Source: CAD feature listing. Evaluate the final solid. Frame: model axes, mm. Coordinates: 2 decimals unless noted, no trailing zeros. Write each loop counter-clockwise with the first axis right and the second up, starting at its lowest first coordinate (ties: lowest second). Pieces come first, ordered by that corner, then holes. Notation, with made-up numbers: M 2,-29.75 L 44,-29.75 A17 ccw 44,-1.75 Z; hole C -26.5,31.25 d10. An arc over 180 degrees is marked long. One line per item, written item: value. Start each with the question number.
Item 1: Pin query (flat end, axial travel): P1, Ø1.5, axis at x = 6.25, z = -0.5, coming from the +Y side. Return the tip coordinate at first contact, or that it passes through.
Item 2: Mould query, pull axis Y, two halves, no side actions, for faces 1 (the cylindrical face through (32.83, 5.67, -1.59)), 2 (the cylindrical face through (-1.14, 3.447, -1.592)), 3 (the flat face through (16, 0, -2)), 4 (the flat face through (0, 5, 0.75)). Classes: released by +Y, released by -Y, zero draft, split by the parting line, or undercut.
Item 3: Cut plane B-B, the plane z = -3.1. Output: boundary loops of the cut face in (x, y).
Item 4: Ray query, L1, parallel to Y at x = -1.5, z = -1.15; L2, parallel to Z at x = 30.25, y = 2.5; L3, parallel to Y at x = 33, z = -3.65. Return the intervals inside material, ascending. Write a range as from..to.
Item 5: Cut plane A-A, the plane z = -0.5. State how many separate pieces and enclosed holes the cut face has, then the cut area to 3 significant figures.
Item 6: Cut plane C-C, the plane x = 33.5. Output: boundary loops of the cut face in (y, z), then the cut area to 3 significant figures.
```python
from build123d import *

# Parameters (mm, degrees)
BOSS_EXTRUDE1_DEPTH = 10
SKETCH4_R           = 1.75
CUT_EXTRUDE2_DEPTH  = 40.100031969


with BuildPart() as part:
    # Sketch1 → Boss-Extrude1 (new body)
    with BuildSketch(Plane(origin=(0, 0, 0), x_dir=(1, 0, 0), z_dir=(0, 1, 0))):
        with BuildLine():
            Line((-5, 4), (-5, -0.75))
            Line((-5, -0.75), (1.104356076, -0.75))
            Line((1.104356076, -0.75), (1.104356076, 0))
            ThreePointArc((1.104356076, 0), (2.25, 1.75), (3.395643924, 0))
            Line((3.395643924, 0), (3.395643924, -0.75))
            Line((3.395643924, -0.75), (5.104356076, -0.75))
            Line((5.104356076, -0.75), (5.104356076, 0))
            ThreePointArc((5.104356076, 0), (6.25, 1.75), (7.395643924, 0))
            Line((7.395643924, 0), (7.395643924, -0.75))
            Line((7.395643924, -0.75), (9.104356076, -0.75))
            Line((9.104356076, -0.75), (9.104356076, 0))
            ThreePointArc((9.104356076, 0), (10.25, 1.75), (11.395643924, 0))
            Line((11.395643924, 0), (11.395643924, -0.75))
            Line((11.395643924, -0.75), (13.104356076, -0.75))
            Line((13.104356076, -0.75), (13.104356076, 0))
            ThreePointArc((13.104356076, 0), (14.25, 1.75), (15.395643924, 0))
            Line((15.395643924, 0), (15.395643924, -0.75))
            Line((15.395643924, -0.75), (17.104356076, -0.75))
            Line((17.104356076, -0.75), (17.104356076, 0))
            ThreePointArc((17.104356076, 0), (18.25, 1.75), (19.395643924, 0))
            Line((19.395643924, 0), (19.395643924, -0.75))
            Line((19.395643924, -0.75), (21.104356076, -0.75))
            Line((21.104356076, -0.75), (21.104356076, 0))
            ThreePointArc((21.104356076, 0), (22.25, 1.75), (23.395643924, 0))
            Line((23.395643924, 0), (23.395643924, -0.75))
            Line((23.395643924, -0.75), (25.104356076, -0.75))
            Line((25.104356076, -0.75), (25.104356076, 0))
            ThreePointArc((25.104356076, 0), (26.25, 1.75), (27.395643924, 0))
            Line((27.395643924, 0), (27.395643924, -0.75))
            Line((27.395643924, -0.75), (29.104356076, -0.75))
            Line((29.104356076, -0.75), (29.104356076, 0))
            ThreePointArc((29.104356076, 0), (30.25, 1.75), (31.395643924, 0))
            Line((31.395643924, 0), (31.395643924, -0.75))
            Line((31.395643924, -0.75), (37.5, -0.75))
            Line((37.5, -0.75), (37.5, 4))
            Line((37.5, 4), (-5, 4))
        make_face()
    extrude(amount=BOSS_EXTRUDE1_DEPTH)

    # Sketch4 → Cut-Extrude2 (cut, through all)
    with BuildSketch(Plane.XY.offset(0.75)):
        with Locations((-1.947821962, 5)):
            Circle(SKETCH4_R)
        with Locations(Location((34.447821962, 5, 0), (0, 0, 180))):
            Circle(SKETCH4_R)
    extrude(amount=-CUT_EXTRUDE2_DEPTH, mode=Mode.SUBTRACT)


solid = part.part
```
From the geometry:
1. P1: passes through
2. face 1: undercut
2. face 2: undercut
2. face 3: released by -Y
2. face 4: zero draft
3. outline: M -5,0 L 37.5,0 L 37.5,10 L -5,10 Z; hole C -1.95,5 d3.5; hole C 34.45,5 d3.5
4. L1: y = 0..3.31, 6.69..10
4. L2: z = -4..-1.75
4. L3: y = 0..4.02, 5.98..10
5. separate pieces: 9
5. enclosed holes: 2
5. area: 206 mm²
6. outline: M 0,-4 L 3.53,-4 L 3.53,0.75 L 0,0.75 Z; M 6.47,-4 L 10,-4 L 10,0.75 L 6.47,0.75 Z
6. area: 33.5 mm²
